```python
from build123d import *

# Parameters (mm, degrees)
IZIM1_R                     = 300
IZIM1_R_2                   = 252.5
Y_KSEKLIK_EKSTR_ZYON1_DEPTH = 30
IZIM2_R                     = 15
KES_EKSTR_ZYON1_DEPTH       = 30


with BuildPart() as part:
    # Çizim1 → Yükseklik-Ekstrüzyon1 (new body)
    with BuildSketch(Plane.XY):
        Circle(IZIM1_R)
        Circle(IZIM1_R_2, mode=Mode.SUBTRACT)
    extrude(amount=Y_KSEKLIK_EKSTR_ZYON1_DEPTH)

    # Çizim2 → Kes-Ekstrüzyon1 (cut)
    with BuildSketch(Plane.XY.offset(30)):
        with Locations((0, 275)):
            Circle(IZIM2_R)
        with Locations((275, 0)):
            Circle(IZIM2_R)
        with Locations((-275, 0)):
            Circle(IZIM2_R)
        with Locations((0, -275)):
            Circle(IZIM2_R)
        with Locations((-144.313707876, -234.090909091)):
            Circle(IZIM2_R)
        with Locations((-234.090909091, -144.313707876)):
            Circle(IZIM2_R)
        with Locations((-234.090909091, 144.313707876)):
            Circle(IZIM2_R)
        with Locations((144.313707876, -234.090909091)):
            Circle(IZIM2_R)
        with Locations((234.090909091, -144.313707876)):
            Circle(IZIM2_R)
        with Locations((234.090909091, 144.313707876)):
            Circle(IZIM2_R)
        with Locations((-144.313707876, 234.090909091)):
            Circle(IZIM2_R)
        with Locations((144.313707876, 234.090909091)):
            Circle(IZIM2_R)
    extrude(amount=-KES_EKSTR_ZYON1_DEPTH, mode=Mode.SUBTRACT)


solid = part.part
```
Can you work these out from the model? Positions are in its coordinate system, mm. Round coordinates to 2 decimals unless told otherwise and drop trailing zeros. Loops run counter-clockwise (first coordinate to the right, second up) from the corner with the lowest first, then second, coordinate; pieces in that order, holes last. Notation, with made-up numbers: M -40,-36.75 L -5,-36.75 A28 cw -5,-1.75 Z; hole C -36.5,-31 d11. An arc over 180 degrees is marked long. Answer as a JSON object with one key per item and string values. Group by question number.
Q1. We'd pull the mould along Y, two halves only. Please class faces 1 (the cylindrical face through (-39.054, 297.447, 14.79)), 2 (the flat face through (-157, 201, 0)), 3 (the cylindrical face through (-245.1, 154.5, 15.2)): +Y half, -Y half, draft (parallel to the pull), parting line (faces both ways), or undercut.
Q2. Imagine slicing it at D-D, the plane z = 15.75. Count the separate pieces of the cut face and the enclosed holes in it, then the cut area to 3 significant figures.
Q3. Imagine slicing it at A-A, the plane y = 0. Please give me the cut outline in (x, z), then the cut area to 3 significant figures.
Q4. Imagine slicing it at B-B, the plane x = -205. Please give me the cut outline in (y, z), then the cut area to 3 significant figures.
Q5. Will these pins go through, and if not, where does the flat tip stop? pin 1 (24 mm diameter, centred on x = 234.09, y = -144.31, fed in from -Z); pin 2 (3 mm diameter, centred on x = 16, z = 8, fed in from +Y); pin 3 (1.5 mm diameter, centred on y = -143.5, z = 25, fed in from -X); pin 4 (6 mm diameter, centred on y = 166, z = 22.5, fed in from -X).
Q6. Imagine slicing it at C-C, the plane y = -275. Please give me the cut outline in (x, z), then the cut area to 3 significant figures.
Q7. Please list where these lines run through material, in increasing order: L1, parallel to Y at x = -154, z = 2.5; L2, parallel to Y at x = 147, z = 14.75; L3, parallel to X at y = -133.5, z = 21.75.
Findings:
{
 "1": {"face 1": "parting line", "face 2": "draft", "face 3": "undercut"},
 "2": {"separate pieces": "1", "enclosed holes": "13", "area": "74,000 mm2"},
 "3": {"outline": "M -300,0 L -290,0 L -290,30 L -300,30 Z; M -260,0 L -252.5,0 L -252.5,30 L -260,30 Z; M 252.5,0 L 260,0 L 260,30 L 252.5,30 Z; M 290,0 L 300,0 L 300,30 L 290,30 Z", "area": "1,050 mm2"},
 "4": {"outline": "M -219.03,0 L -147.42,0 L -147.42,30 L -219.03,30 Z; M 147.42,0 L 219.03,0 L 219.03,30 L 147.42,30 Z", "area": "4,300 mm2"},
 "5": {"pin 1": "passes through", "pin 2": "stops at y = 299.65", "pin 3": "stops at x = -263.86", "pin 4": "stops at x = -251.86"},
 "6": {"outline": "M -119.9,0 L -15,0 L -15,30 L -119.9,30 Z; M 15,0 L 119.9,0 L 119.9,30 L 15,30 Z", "area": "6,290 mm2"},
 "7": {"L1": "y = -257.46 to -245.54, -222.64 to -200.1, 200.1 to 222.64, 245.54 to 257.46", "L2": "y = -261.52 to -248.85, -219.33 to -205.3, 205.3 to 219.33, 248.85 to 261.52", "L3": "x = -268.66 to -244.49, -223.7 to -214.32, 214.32 to 223.7, 244.49 to 268.66"}
}
